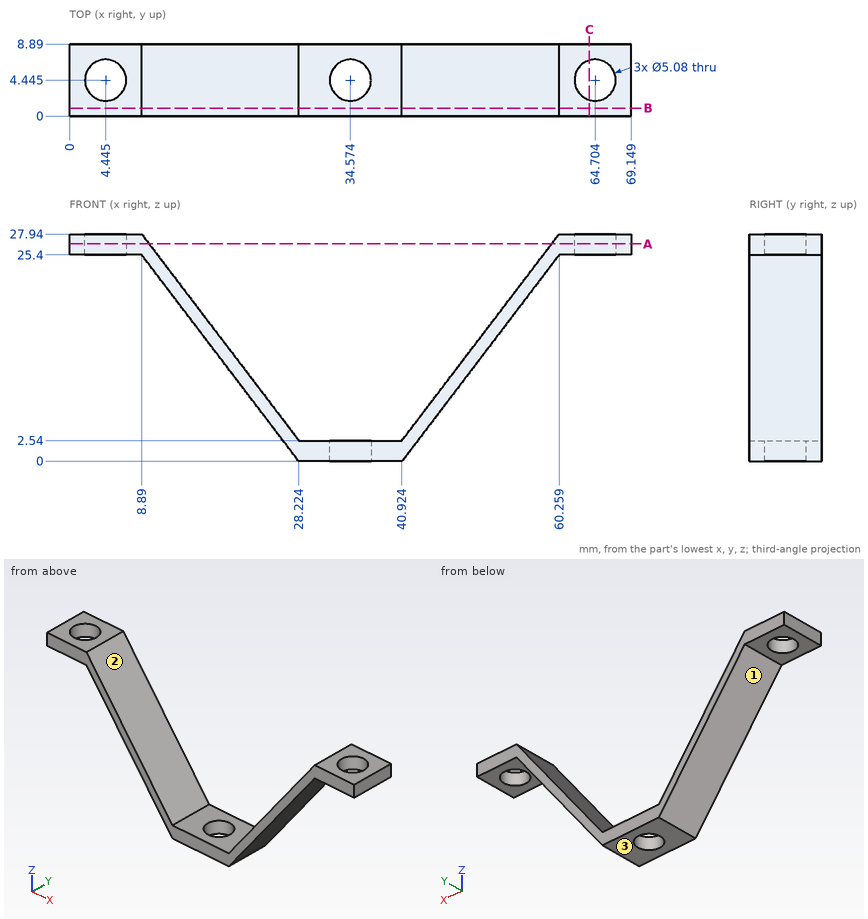
Job drawing, mm, ordinate dimensions from the low corner. One solid piece. Give positions to 0.01 mm unless a question says otherwise; leave off trailing zeros. Loops run counter-clockwise (first coordinate to the right, second up) from the corner with the lowest first, then second, coordinate; pieces in that order, holes last. Notation, with made-up numbers: (-11.5, 53) -> (22.5, 53) arc R10 cw to (22.5, 59) -> close; hole circle Ø6 at (-17, -20). An arc over 180 degrees is marked (long way). Use a Markdown table: item, result. Add a question column.
(1) Slice it at C-C on x = 64. List the corners of the cut face in (y, z) (1 decimal), and give its area (3 significant figures).
(2) Wall check: line 1 along Z through (x, y) = (29, 3); line 2 along Z through (x, y) = (62, 6.5); line 3 along X through (y, z) = (8, 21) (1 decimal). Give the ranges that are in metal, low to high.
(3) Mould opens along X. For the marked faces 1, 2 and 3 say: +X half, -X half, draft (parallel to the pull), parting line (faces both ways), or undercut.
(4) Slice it at A-A on z = 26.75. List the corners of the cut face in (x, y) (1 decimal).
(5) Slice it at B-B on y = 1. List the corners of the cut face in (x, z) (1 decimal).
(6) Drop flat-ended pins along their axis: pin 1 Ø5 at (x, y) = (44.5, 2.5) entering from +Z; pin 2 Ø1.5 at (x, y) = (49.5, 7) entering from +Z; pin 3 Ø5 at (x, y) = (19, 2) entering from -Z (1 decimal). Give the stop position or say it passes through.
Filled sheet:
| question | item | result |
|---|---|---|
| 1 | outline | (0, 25.4) -> (2, 25.4) -> (2, 27.9) -> (0, 27.9) -> close; (6.9, 25.4) -> (8.9, 25.4) -> (8.9, 27.9) -> (6.9, 27.9) -> close |
| 1 | area | 10.2 mm2 |
| 2 | line 1 | 0 to 2.54 |
| 2 | line 2 | 25.4 to 27.94 |
| 2 | line 3 | 12.2 to 14.2, 55 to 56.9 |
| 3 | face 1 | -X half |
| 3 | face 2 | undercut |
| 3 | face 3 | draft |
| 4 | outline | (0, 0) -> (9.8, 0) -> (9.8, 8.9) -> (0, 8.9) -> close; (59.4, 0) -> (69.1, 0) -> (69.1, 8.9) -> (59.4, 8.9) -> close; hole circle Ø5.1 at (4.4, 4.4); hole circle Ø5.1 at (64.7, 4.4) |
| 5 | outline | (0, 25.4) -> (8.9, 25.4) -> (28.2, 0) -> (40.9, 0) -> (60.3, 25.4) -> (69.1, 25.4) -> (69.1, 27.9) -> (60.3, 27.9) -> (40.9, 2.5) -> (28.2, 2.5) -> (8.9, 27.9) -> (0, 27.9) -> close |
| 6 | pin 1 | z = 10.52 |
| 6 | pin 2 | z = 14.79 |
| 6 | pin 3 | z = 8.8 |
